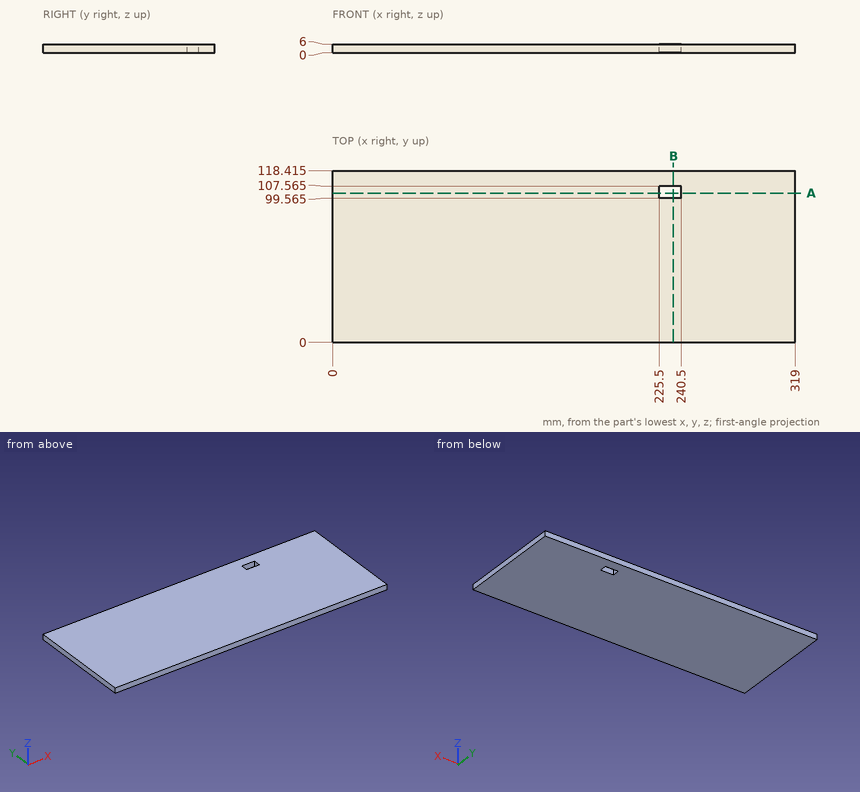
Geometry check sheet. Reference: drawing and pictorial views, mm from the part's lowest x, y, z. Coordinates: 2 decimals unless noted, no trailing zeros. Write each loop counter-clockwise with the first axis right and the second up, starting at its lowest first coordinate (ties: lowest second). Pieces come first, ordered by that corner, then holes. Notation, with made-up numbers: M -38,24 L 3,24 A20 cw 3,37 Z; hole C 29,26.5 d3. An arc over 180 degrees is marked long. One line per question, with ' | ' between items.
1) Sectioned sample at B-B on x = 235. Record the cut outline in (y, z) (3 decimals).
Solutions:
outline: M 0,0 L 99.565,0 L 99.565,6 L 0,6 Z; M 107.565,0 L 118.415,0 L 118.415,6 L 107.565,6 Z
2) Sectioned sample at A-A on y = 103. Record the cut outline in (x, z), then the cut area to 3 significant figures.
Solutions:
outline: M 0,0 L 225.5,0 L 225.5,6 L 0,6 Z; M 240.5,0 L 319,0 L 319,6 L 240.5,6 Z | area: 1,820 mm^2
3) Material ranges on L1, parallel to Y at x = 228, z = 2.4 (3 decimals); L2, parallel to X at y = 102, z = 0.8, recorded low to high.
Solutions:
L1: 0 to 99.565, 107.565 to 118.415 | L2: 0 to 225.5, 240.5 to 319
